Input: part model. Units: mm. Frame: model coordinates. A direction names the side the tool comes from. Coordinates: 2 decimals unless noted, no trailing zeros. Loops run counter-clockwise (first coordinate to the right, second up) from the corner with the lowest first, then second, coordinate; pieces in that order, holes last.
```python
from build123d import *

# Parameters (mm, degrees)
SKETCH_1_R          = 21
EXTRUDE_1_DEPTH     = 10
SKETCH_4_R          = 20
EXTRUDE_3_DEPTH     = 16
SKETCH_6_R          = 1.5
CUT_EXTRUDE_1_DEPTH = 4
SKETCH_7_R          = 10
SKETCH_7_R_2        = 9
EXTRUDE_4_DEPTH     = 1.5
SKETCH_8_W          = 20
SKETCH_8_H          = 6
CUT_EXTRUDE_2_DEPTH = 5


with BuildPart() as part:
    # 草图1 → 凸台-拉伸1 (new body)
    with BuildSketch(Plane(origin=(0, 0, 0), x_dir=(1, 0, 0), z_dir=(0, 1, 0))):
        Circle(SKETCH_1_R)
    extrude(amount=EXTRUDE_1_DEPTH)

    # 草图4 → 凸台-拉伸3 (add)
    with BuildSketch(Plane(origin=(0, 10, 0), x_dir=(1, 0, 0), z_dir=(0, 1, 0))):
        Circle(SKETCH_4_R)
    extrude(amount=EXTRUDE_3_DEPTH)

    # 草图6 → 切除-拉伸1 (cut)
    with BuildSketch(Plane.XZ):
        with Locations((12.727922061, 12.727922061)):
            Circle(SKETCH_6_R)
        with Locations((12.727922061, -12.727922061)):
            Circle(SKETCH_6_R)
        with Locations((-12.727922061, -12.727922061)):
            Circle(SKETCH_6_R)
        with Locations((-12.727922061, 12.727922061)):
            Circle(SKETCH_6_R)
    extrude(amount=-CUT_EXTRUDE_1_DEPTH, mode=Mode.SUBTRACT)

    # 草图7 → 凸台-拉伸4 (add)
    with BuildSketch(Plane.XZ):
        Circle(SKETCH_7_R)
        Circle(SKETCH_7_R_2, mode=Mode.SUBTRACT)
    extrude(amount=EXTRUDE_4_DEPTH)

    # 草图8 → 切除-拉伸2 (cut)
    with BuildSketch(Plane.XY.offset(21)):
        with Locations((0, 4)):
            Rectangle(SKETCH_8_W, SKETCH_8_H)
    extrude(amount=-CUT_EXTRUDE_2_DEPTH, mode=Mode.SUBTRACT)


solid = part.part
```
Item 1: Section query C-C (y = 15.75). Output: boundary loops of the cut face in (x, z), then the cut area to 3 significant figures.
Result:
outline: circle Ø40 at (0, 0)
area: 1,260 mm2
Item 2: Contact query for flat-ended pins moving along their axis: P1, Ø12, axis at x = -10, y = 23, coming from the -Z side; P2, Ø8, axis at y = 23, z = 4, coming from the -X side; P3, Ø6, axis at y = 15.5, z = -3.5, coming from the +X side; P4, Ø3, axis at x = 15.5, z = 16.5, coming from the -Y side. Output: stop coordinate, or through.
Result:
P1: stops at z = -19.6
P2: stops at x = -20
P3: stops at x = 19.99
P4: passes through
Item 3: Section query B-B (x = 0). Output: boundary loops of the cut face in (y, z).
Result:
outline: (-1.5, -10) - (0, -10) - (0, -21) - (10, -21) - (10, -20) - (26, -20) - (26, 20) - (10, 20) - (10, 21) - (7, 21) - (7, 16) - (1, 16) - (1, 21) - (0, 21) - (0, 10) - (-1.5, 10) - (-1.5, 9) - (0, 9) - (0, -9) - (-1.5, -9) - close
Item 4: Reachability of faces 1 (the face through (-4.336, 17.888, 19.524)), 2 (the face through (-13, 4, 13)), 3 (the face through (10, 4, 17)) from +Z, -Z, +X, -X, +Y, -Y: full face, straight path, thin tool, end or side. Return the list, or none.
Result:
face 1: +Y
face 2: -Y
face 3: +Z
Item 5: Section query A-A (z = 0). Output: boundary loops of the cut face in (x, y).
Result:
outline: (-21, 0) - (-10, 0) - (-10, -1.5) - (-9, -1.5) - (-9, 0) - (9, 0) - (9, -1.5) - (10, -1.5) - (10, 0) - (21, 0) - (21, 10) - (20, 10) - (20, 26) - (-20, 26) - (-20, 10) - (-21, 10) - close
Item 6: Line query: L1, parallel to Y at x = 4, z = 18; L2, parallel to Z at x = 0, y = -1; L3, parallel to Y at x = 13, z = -10.5. Output: solid intervals per line, ascending.
Result:
L1: y = 0 to 1, 7 to 26
L2: z = -10 to -9, 9 to 10
L3: y = 0 to 26
Item 7: Mould query, pull axis X, two halves, no side actions, for faces 4 (the face through (-2.73, 4.93, -20.82)), 5 (the face through (0, 26, 0)), 6 (the face through (14.16, 1.97, -12.28)), 7 (the face through (-12.92, 1.97, -11.24)). Classes: +X half, -X half, draft (parallel to the pull), parting line (faces both ways), or undercut.
Result:
face 4: parting line
face 5: draft
face 6: undercut
face 7: undercut
Item 8: Section query D-D (z = -8). Output: boundary loops of the cut face in (x, y), then the cut area to 3 significant figures.
Result:
outline: (-19.42, 0) - (-6, 0) - (-6, -1.5) - (-4.12, -1.5) - (-4.12, 0) - (4.12, 0) - (4.12, -1.5) - (6, -1.5) - (6, 0) - (19.42, 0) - (19.42, 10) - (18.33, 10) - (18.33, 26) - (-18.33, 26) - (-18.33, 10) - (-19.42, 10) - close
area: 981 mm2
